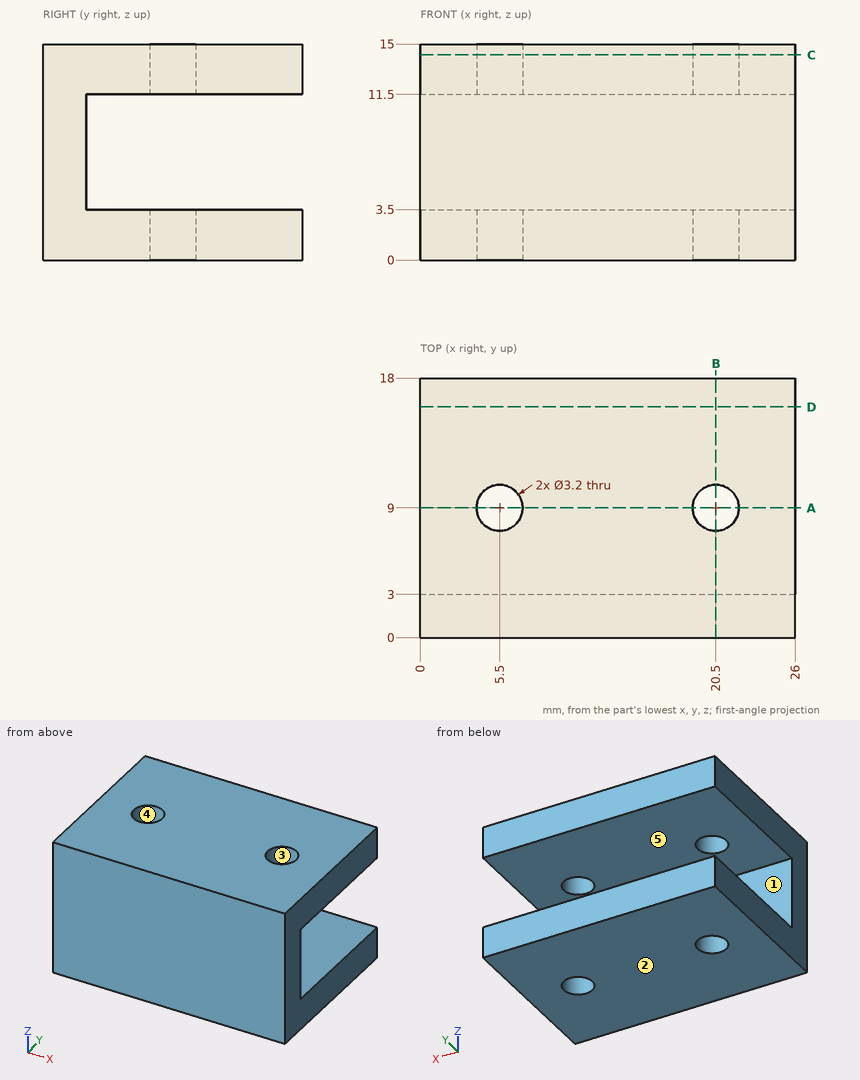
Job drawing, mm, ordinate dimensions from the low corner. One solid piece. A direction names the side the tool comes from. Give positions to 0.01 mm unless a question says otherwise; leave off trailing zeros. Order: outer loops, then holes, each group sorted by start corner. A loop starts at its lowest first (then second) coordinate and runs counter-clockwise, first axis right, second up. Notation, with made-up numbers: (-14, -5) - (31, -5) arc R16 ccw to (31, 11) - close; hole circle Ø1 at (55, 10). An arc over 180 degrees is marked (long way). Return JSON: item names as keys, results as strings.
1) Cut at A-A, the plane y = 9. Give the cut face in (x, z).
Geometry says:
{"outline": "(0, 0) - (3.9, 0) - (3.9, 3.5) - (0, 3.5) - close; (0, 11.5) - (3.9, 11.5) - (3.9, 15) - (0, 15) - close; (7.1, 0) - (18.9, 0) - (18.9, 3.5) - (7.1, 3.5) - close; (7.1, 11.5) - (18.9, 11.5) - (18.9, 15) - (7.1, 15) - close; (22.1, 0) - (26, 0) - (26, 3.5) - (22.1, 3.5) - close; (22.1, 11.5) - (26, 11.5) - (26, 15) - (22.1, 15) - close"}
2) Flat gauge pins, fed straight in: P1, Ø1.9, axis at x = 5.5, y = 9, coming from the +Z side; P2, Ø4, axis at x = 6.5, z = 9, coming from the +Y side. Where does each tip first touch, or does it go through?
Geometry says:
{"P1": "through", "P2": "y = 3"}
3) 3-axis set-ups, long thin cutter, end or side, ignore diameter. For the marked faces 4 and 5: which of +Z, -Z, +X, -X, +Y, -Y reach the whole face in a straight line?
Geometry says:
{"face 4": "+Z, -Z", "face 5": "+X, -X, +Y"}
4) Cut at D-D, the plane y = 16. Give the cut face in (x, z).
Geometry says:
{"outline": "(0, 0) - (26, 0) - (26, 3.5) - (0, 3.5) - close; (0, 11.5) - (26, 11.5) - (26, 15) - (0, 15) - close"}
5) Cut at C-C, the plane z = 14.25. Give the cut face in (x, y).
Geometry says:
{"outline": "(0, 0) - (26, 0) - (26, 18) - (0, 18) - close; hole circle Ø3.2 at (5.5, 9); hole circle Ø3.2 at (20.5, 9)"}
6) Pull direction Z, two halves, no side cores. Call the marked faces 1, 2 and 3: pulls with the +Z half, pulls with the -Z half, needs draft (parallel to the pull), parting line crosses it, or undercut.
Geometry says:
{"face 1": "undercut", "face 2": "pulls with the -Z half", "face 3": "needs draft"}
7) Cut at B-B, the plane x = 20.5. Give the cut face in (y, z), plus the area to 3 significant figures.
Geometry says:
{"outline": "(0, 0) - (7.4, 0) - (7.4, 3.5) - (3, 3.5) - (3, 11.5) - (7.4, 11.5) - (7.4, 15) - (0, 15) - close; (10.6, 0) - (18, 0) - (18, 3.5) - (10.6, 3.5) - close; (10.6, 11.5) - (18, 11.5) - (18, 15) - (10.6, 15) - close", "area": "128 mm²"}
8) Probe line 1 (X direction, y = 9, z = 2.3); line 2 (Y direction, x = 5.5, z = 2.7); line 3 (Z direction, x = 20, y = 4.25). List the from-to ranges inside material, lowest first. Write a range as from..to.
Geometry says:
{"line 1": "0..3.9, 7.1..18.9, 22.1..26", "line 2": "0..7.4, 10.6..18", "line 3": "0..3.5, 11.5..15"}
